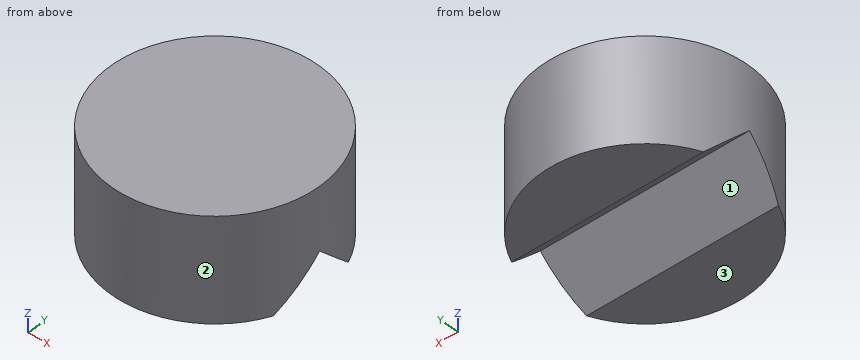
from build123d import *

# Parameters (mm, degrees)
F0_R     = 6.35
F1_DEPTH = 6.35
F2_R     = 1.27
F7_DEPTH = 12.7


with BuildPart() as f1:
    # F0 (on Top) → F1 (new body)
    with BuildSketch(Plane.XY):
        Circle(F0_R)
    extrude(amount=F1_DEPTH)

    # F2 (on Top) → F5 section 0
    with BuildSketch(Plane.XY, mode=Mode.PRIVATE) as f5_s0:
        Circle(F2_R)
    loft([Vertex(0, 0, -2.54), f5_s0.sketch], mode=Mode.SUBTRACT)

    # F6 (on Right) → F7 (cut, symmetric)
    with BuildSketch(Plane.YZ):
        Polygon((0, -2.54), (2.54, 0), (0, 2.54), (-2.54, 0), align=None)
    extrude(amount=F7_DEPTH, both=True, mode=Mode.SUBTRACT)


solid = f1.part
Verification items for the finished model (mm, model axes). Face numbers are marked on the shaded views. Round coordinates to 2 decimals unless told otherwise and drop trailing zeros. Loops run counter-clockwise (first coordinate to the right, second up) from the corner with the lowest first, then second, coordinate; pieces in that order, holes last. Notation, with made-up numbers: (23, 86.5) - (37, 86.5) arc R14 cw to (37, 110.5) - close; hole circle Ø9 at (81, 65.25). An arc over 180 degrees is marked (long way). Use a Markdown table: item, result. Add a question column.
1. Thickness scan on probe 1 along Y at (x, z) = (1, 0.75); probe 2 along Y at (x, z) = (-5, 0.5); probe 3 along Y at (x, z) = (-2.75, 4.5). Record the ranges inside material, lowest first. Write a range as [from, to].
2. Release check for a two-part mould opening along Y. For the marked faces 1, 2 and 3 record: released by +Y, released by -Y, zero draft, split by the parting line, or undercut.
3. Section check D-D, the plane x = 3.25. Record the boundary of the cut face in (y, z).
4. Gauge pin test, flat end, axial feed: pin 1 (3 mm diameter, centred on x = -4, y = 0.5, fed in from -Z). Record the tip position at first contact, or that the pin passes through.
5. Section check B-B, the plane z = 3.5. Record the boundary of the cut face in (x, y).
6. Section check C-C, the plane y = 0.5. Record the boundary of the cut face in (x, z), plus the area to 3 significant figures.
7. Section check A-A, the plane x = 0. Record the boundary of the cut face in (y, z).
Checks:
| question | item | result |
|---|---|---|
| 1 | probe 1 | y = [-6.27, -1.79], [1.79, 6.27] |
| 1 | probe 2 | y = [-3.91, -2.04], [2.04, 3.91] |
| 1 | probe 3 | y = [-5.72, 5.72] |
| 2 | face 1 | undercut |
| 2 | face 2 | split by the parting line |
| 2 | face 3 | zero draft |
| 3 | outline | (-5.46, 0) - (-2.54, 0) - (0, 2.54) - (2.54, 0) - (5.46, 0) - (5.46, 6.35) - (-5.46, 6.35) - close |
| 4 | pin 1 | stops at z = 0.54 |
| 5 | outline | circle Ø12.7 at (0, 0) |
| 6 | outline | (-6.33, 2.04) - (6.33, 2.04) - (6.33, 6.35) - (-6.33, 6.35) - close |
| 6 | area | 54.6 mm^2 |
| 7 | outline | (-6.35, 0) - (-2.54, 0) - (0, 2.54) - (2.54, 0) - (6.35, 0) - (6.35, 6.35) - (-6.35, 6.35) - close |
